```python
from build123d import *

# Parameters (mm, degrees)
SKETCH2_W           = 106
SKETCH2_H           = 67.7
BOSS_EXTRUDE1_DEPTH = 8.4
BOSS_EXTRUDE2_DEPTH = 1
SKETCH5_W           = 95.04
SKETCH5_H           = 53.86
CUT_EXTRUDE1_DEPTH  = 0.1


with BuildPart() as part:
    # Sketch2 → Boss-Extrude1 (new body)
    with BuildSketch(Plane(origin=(0, 0, 0), x_dir=(1, 0, 0), z_dir=(0, 1, 0))):
        Rectangle(SKETCH2_W, SKETCH2_H)
    extrude(amount=BOSS_EXTRUDE1_DEPTH)

    # Sketch3 → Boss-Extrude2 (add)
    with BuildSketch(Plane(origin=(0, 8.4, 0), x_dir=(1, 0, 0), z_dir=(0, 1, 0))):
        with BuildLine():
            Line((-55.5, 43.85), (55.5, 43.85))
            ThreePointArc((55.5, 43.85), (59.742640687, 42.092640687), (61.5, 37.85))
            Line((61.5, 37.85), (61.5, -34.65))
            ThreePointArc((61.5, -34.65), (59.742640687, -38.892640687), (55.5, -40.65))
            Line((55.5, -40.65), (-55.5, -40.65))
            ThreePointArc((-55.5, -40.65), (-59.742640687, -38.892640687), (-61.5, -34.65))
            Line((-61.5, -34.65), (-61.5, 37.85))
            ThreePointArc((-61.5, 37.85), (-59.742640687, 42.092640687), (-55.5, 43.85))
        make_face()
    extrude(amount=-BOSS_EXTRUDE2_DEPTH)

    # Sketch5 → Cut-Extrude1 (cut)
    with BuildSketch(Plane(origin=(0, 8.4, 0), x_dir=(1, 0, 0), z_dir=(0, 1, 0))):
        with Locations((0, 1.6)):
            Rectangle(SKETCH5_W, SKETCH5_H)
    extrude(amount=-CUT_EXTRUDE1_DEPTH, mode=Mode.SUBTRACT)


solid = part.part
```
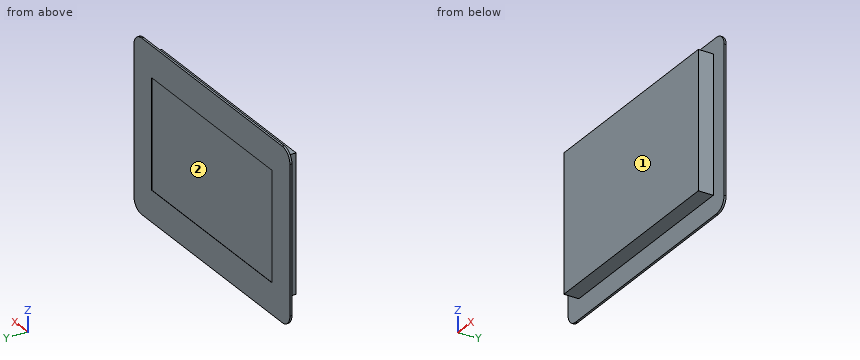
Could you check a few things on this model? Use its own coordinates, in mm. Face numbers are marked on the shaded views. Round coordinates to 2 decimals unless told otherwise and drop trailing zeros. Loops run counter-clockwise (first coordinate to the right, second up) from the corner with the lowest first, then second, coordinate; pieces in that order, holes last. Notation, with made-up numbers: (80, 7) - (100, 7) arc R19 ccw to (100, 24) - close; hole circle Ø2 at (81.5, -33). An arc over 180 degrees is marked (long way). Use CSV: the item, a comma, the result in double quotes.
Item 1: Will these pins go through, and if not, where does the flat tip stop? pin 1 (1.5 mm diameter, centred on y = 1.5, z = 2, fed in from +X); pin 2 (2 mm diameter, centred on x = -18, y = 2, fed in from +Z); pin 3 (1.5 mm diameter, centred on y = 4.5, z = -28.5, fed in from -X).
Here are the results:
pin 1,"stops at x = 53"
pin 2,"stops at z = 33.85"
pin 3,"stops at x = -53"
Item 2: If we section it at C-C on y = 3: List the corners of the cut face in (x, z) for me.
Here are the results:
outline,"(-53, -33.85) - (53, -33.85) - (53, 33.85) - (-53, 33.85) - close"
Item 3: If we mould it in two halves opening along X, with no side actions, what happens to the marked faces 1 and 2? For each: pulls with the +X half, pulls with the -X half, needs draft (parallel to the pull), parting line crosses it, or undercut.
Here are the results:
face 1,"needs draft"
face 2,"undercut"
Item 4: If we section it at D-D on z = -15.5: List the corners of the cut face in (x, y) for me, then the cut area to 3 significant figures.
Here are the results:
outline,"(-61.5, 7.4) - (-53, 7.4) - (-53, 0) - (53, 0) - (53, 7.4) - (61.5, 7.4) - (61.5, 8.4) - (47.52, 8.4) - (47.52, 8.3) - (-47.52, 8.3) - (-47.52, 8.4) - (-61.5, 8.4) - close"
area,"898 mm²"
Item 5: If we section it at B-B on x = 19: List the corners of the cut face in (y, z) for me, then the cut area to 3 significant figures.
Here are the results:
outline,"(0, -33.85) - (7.4, -33.85) - (7.4, -43.85) - (8.4, -43.85) - (8.4, -28.53) - (8.3, -28.53) - (8.3, 25.33) - (8.4, 25.33) - (8.4, 40.65) - (7.4, 40.65) - (7.4, 33.85) - (0, 33.85) - close"
area,"580 mm²"
Item 6: If we section it at A-A on z = -32.5: List the corners of the cut face in (x, y) for me.
Here are the results:
outline,"(-61.5, 7.4) - (-53, 7.4) - (-53, 0) - (53, 0) - (53, 7.4) - (61.5, 7.4) - (61.5, 8.4) - (-61.5, 8.4) - close"
Item 7: I need wall thicknesses on L1, parallel to Y at x = 4.5, z = 12.5; L2, parallel to Z at x = -48, y = 2.75; L3, parallel to X at y = 5.25, z = -30.5. Which ranges of each line are inside material? Lowest first, please. Write a range as [from, to].
Here are the results:
L1,"y = [0, 8.3]"
L2,"z = [-33.85, 33.85]"
L3,"x = [-53, 53]"
